from build123d import *

# Parameters (mm, degrees)
BOSS_EXTRUDE1_DEPTH         = 76.2
F_3_8_1_75_DIAMETER_HOLE1_D = 44.45
TAP_DRILL_FOR_3_8_24_TAP1_D = 8.4328
TAP_DRILL_FOR_3_8_24_TAP2_D = 12.7


with BuildPart() as part:
    # Sketch1 → Boss-Extrude1 (new body)
    with BuildSketch(Plane.XY):
        Polygon((0, 0), (0, 38.1), (177.8, 38.1), (177.8, 0), (165.1, 0), (165.1, 25.4), (12.7, 25.4), (12.7, 0), align=None)
    extrude(amount=BOSS_EXTRUDE1_DEPTH)

    # 3/8 (1.75) Diameter Hole1 (through all)
    with Locations(Plane(origin=(0, 38.1, 0), x_dir=(1, 0, 0), z_dir=(0, 1, 0))):
        with Locations((88.9, -38.1)):
            Hole(F_3_8_1_75_DIAMETER_HOLE1_D / 2)

    # Tap Drill for 3/8-24 Tap1 (through all)
    with Locations(Plane(origin=(0, 38.1, 0), x_dir=(1, 0, 0), z_dir=(0, 1, 0))):
        with Locations((44.45, -38.1), (133.35, -38.1)):
            Hole(TAP_DRILL_FOR_3_8_24_TAP1_D / 2)

    # Tap Drill for 3/8-24 Tap2 (through all)
    with Locations(Plane(origin=(177.8, 0, 0), x_dir=(0, 0, -1), z_dir=(1, 0, 0))):
        with Locations((-57.15, 12.7), (-19.05, 12.7)):
            Hole(TAP_DRILL_FOR_3_8_24_TAP2_D / 2)


solid = part.part
Can you work these out from the model? Positions are in its coordinate system, mm. A direction names the side the tool comes from. Give positions to 0.01 mm unless a question says otherwise; leave off trailing zeros. Loops run counter-clockwise (first coordinate to the right, second up) from the corner with the lowest first, then second, coordinate; pieces in that order, holes last. Notation, with made-up numbers: M -12.75,4 L 19.25,4 A22 cw 19.25,40 Z; hole C 7.25,55 d2. An arc over 180 degrees is marked long. One line per item, written item: value. Start each with the question number.
1) If we section it at D-D, the plane y = 12.7: Write out the boundary of the cut face in (x, z).
2) If we section it at A-A, the plane x = 44.45: Write out the boundary of the cut face in (y, z).
3) If I drill on line 1 (Z direction, x = 9, y = 12); line 2 (X direction, y = 31, z = 38); line 3 (Y direction, x = 4, z = 57), over which ranges is the centre line in solid material (lowest first)? Write a range as [from, to].
4) On a 3-axis mill with a long thin cutter (end or side, diameter ignored), from which of +Z, -Z, +X, -X, +Y, -Y can I reach the whole of each face in a straight line? I mean faces 1 (the face through (73, 25.4, 54)), 2 (the face through (171.36, 16.99, 52.47)). Say none if no direction works.
5) If we section it at B-B, the plane y = 2.5: Write out the boundary of the cut face in (x, z).
6) If we section it at C-C, the plane z = 38.1: Write out the boundary of the cut face in (x, y) (3 decimals), and give its area (3 significant figures).
7) I'm going to push flat-ended pins straight in: pin 1 (7.5 mm diameter, centred on x = 44.45, z = 38.1, fed in from +Y); pin 2 (10 mm diameter, centred on x = 58, z = 62, fed in from -Y). Where does each tip first touch, or does it pass through?
8) Thinking about a two-plate mould opening in Z: for faces 3 (the face through (172, 0, 38)), 4 (the face through (90, 28, 0)), 5 (the face through (136.5, 31.7, 35.3)), which applies, +Z half, -Z half, draft (parallel to the pull), parting line (faces both ways), or undercut?
Completed:
1. outline: M 0,0 L 12.7,0 L 12.7,12.7 L 0,12.7 Z; M 0,25.4 L 12.7,25.4 L 12.7,50.8 L 0,50.8 Z; M 0,63.5 L 12.7,63.5 L 12.7,76.2 L 0,76.2 Z; M 165.1,0 L 177.8,0 L 177.8,12.7 L 165.1,12.7 Z; M 165.1,25.4 L 177.8,25.4 L 177.8,50.8 L 165.1,50.8 Z; M 165.1,63.5 L 177.8,63.5 L 177.8,76.2 L 165.1,76.2 Z
2. outline: M 25.4,0 L 38.1,0 L 38.1,33.88 L 25.4,33.88 Z; M 25.4,42.32 L 38.1,42.32 L 38.1,76.2 L 25.4,76.2 Z
3. line 1: z = [0, 12.74], [25.36, 50.84], [63.46, 76.2]
3. line 2: x = [0, 40.23], [48.67, 66.68], [111.12, 129.13], [137.57, 177.8]
3. line 3: y = [0, 6.35], [19.05, 38.1]
4. face 1: +Z, -Z, -Y
4. face 2: +X, -X
5. outline: M 0,0 L 12.7,0 L 12.7,76.2 L 0,76.2 Z; M 165.1,0 L 177.8,0 L 177.8,76.2 L 165.1,76.2 Z
6. outline: M 0,0 L 12.7,0 L 12.7,25.4 L 40.234,25.4 L 40.234,38.1 L 0,38.1 Z; M 48.666,25.4 L 66.675,25.4 L 66.675,38.1 L 48.666,38.1 Z; M 111.125,25.4 L 129.134,25.4 L 129.134,38.1 L 111.125,38.1 Z; M 137.566,25.4 L 165.1,25.4 L 165.1,0 L 177.8,0 L 177.8,38.1 L 137.566,38.1 Z
6. area: 2,120 mm^2
7. pin 1: passes through
7. pin 2: stops at y = 25.4
8. face 3: draft
8. face 4: -Z half
8. face 5: undercut
